Work out the finished part from the listing and answer in its coordinate system (mm). A direction names the side the tool comes from. Coordinates: 2 decimals unless noted, no trailing zeros. Order: outer loops, then holes, each group sorted by start corner. A loop starts at its lowest first (then second) coordinate and runs counter-clockwise, first axis right, second up. Notation, with made-up numbers: (64, -17.5) -> (123, -17.5) arc R12 ccw to (123, 2.5) -> close; hole circle Ø4 at (-27.75, 16). An arc over 180 degrees is marked (long way). Use one line per item in the form item = value.
Autodesk Inventor part; units mm, degrees
ref_plane "YZ Plane" through (0, 0, 0) normal (1, 0, 0) x (0, 1, 0)
ref_plane "XZ Plane" through (0, 0, 0) normal (0, 1, 0) x (-1, 0, 0)
ref_plane "XY Plane" through (0, 0, 0) normal (0, 0, 1) x (1, 0, 0)
sketch "Sketch1: base" plane through (0, 0, 0) normal (0, 0, 1) x (1, 0, 0)
  circle A0 centre (0, 0) radius 18
  line L0 (4.45, -17.4413) -> (4.45, -27.4413)
  line L1 (4.45, -27.4413) -> (-4.45, -27.4413)
  line L2 (-4.45, -27.4413) -> (-4.45, -17.4413)
  line L3 (-2.45, -22.3413) -> (2.45, -22.3413)
  line L4 (2.45, -22.3413) -> (2.45, -25.4413)
  line L5 (2.45, -25.4413) -> (-2.45, -25.4413)
  line L6 (-2.45, -25.4413) -> (-2.45, -22.3413)
  line L7 (-2, -22.2913) -> (2, -22.2913) construction
  line L8 (2, -25.4913) -> (-2, -25.4913) construction
  arc A1 (-2, -22.2913) -> (-2, -25.4913) centre (-0.0791, -23.8913) ccw construction
  arc A2 (2, -25.4913) -> (2, -22.2913) centre (0.0791, -23.8913) ccw construction
  point P0 (0, -22.3413)
  point P1 (0, -27.4413)
  point P2 (0, -22.2913)
  point P3 (-2.45, -23.8913)
  dimension "door_diameter" = 36
  dimension "axle_width" = 4.9
  dimension "axle_height" = 3.1
  dimension "handle_height" = 10
  dimension "spacing_height" = 2
  dimension "spacing_width" = 2
  dimension "d14" = 4
  dimension "d16" = 3.2
  dimension "d17" = 2.5
sketch "Sketch2: text" plane through (0, 0, 0) normal (0, 0, 1) x (1, 0, 0)
  line L0 (-1.5, -16.3413) -> (1.5, -16.3413) construction
  line L1 (1.5, -16.3413) -> (1.5, -19.3413) construction
  line L2 (1.5, -19.3413) -> (-1.5, -19.3413) construction
  line L3 (-1.5, -19.3413) -> (-1.5, -16.3413) construction
  line L4 (4.45, -27.4413) -> (-4.45, -27.4413) construction
  line L5 (-4.45, -27.4413) -> (-4.45, -17.4413) construction
  line L6 (4.45, -17.4413) -> (4.45, -27.4413) construction
  line L7 (-2.45, -22.3413) -> (2.45, -22.3413) construction
  line L8 (2.45, -22.3413) -> (2.45, -25.4413) construction
  line L9 (-2.45, -25.4413) -> (-2.45, -22.3413) construction
  line L10 (2.45, -25.4413) -> (-2.45, -25.4413) construction
  circle A0 centre (0, 0) radius 18 construction
  line L11 (-2.7183, -17.1558) -> (-1.8376, -17.1558)
  line L12 (-1.8376, -17.1558) -> (-1.4061, -18.5561)
  line L13 (-1.4061, -18.5561) -> (-0.9628, -17.1558)
  line L14 (-0.9628, -17.1558) -> (-0.1086, -17.1558)
  line L15 (-0.1086, -17.1558) -> (-1.048, -19.3663)
  line L16 (-1.048, -19.3663) -> (-1.7995, -19.3663)
  line L17 (-1.7995, -19.3663) -> (-2.7183, -17.1558)
  line L18 (0.8777, -17.1969) -> (0.0763, -17.0531)
  spline S0 degree 2 poles (0.0763, -17.0531) (0.1761, -16.6715) (0.7427, -16.2634) (1.2623, -16.2634) knots 0 0 0 1 2 2 2
  spline S1 degree 2 poles (1.2623, -16.2634) (1.8611, -16.2634) (2.3924, -16.7096) (2.3924, -17.0443) knots 0 0 0 1 2 2 2
  spline S2 degree 2 poles (2.3924, -17.0443) (2.3924, -17.2439) (2.1752, -17.5639) (1.9551, -17.6842) knots 0 0 0 1 2 2 2
  spline S3 degree 2 poles (1.9551, -17.6842) (2.1341, -17.7282) (2.2281, -17.787) knots 0 0 0 1 1 1
  spline S4 degree 2 poles (2.2281, -17.787) (2.3807, -17.8809) (2.548, -18.1862) (2.548, -18.3975) knots 0 0 0 1 2 2 2
  spline S5 degree 2 poles (2.548, -18.3975) (2.548, -18.6647) (2.2692, -19.1549) (1.7466, -19.4191) (1.318, -19.4191) knots 0 0 0 1 2 3 3 3
  spline S6 degree 2 poles (1.318, -19.4191) (0.9041, -19.4191) (0.4227, -19.2224) (0.1115, -18.8467) (0.0294, -18.5619) knots 0 0 0 1 2 3 3 3
  line L19 (0.0294, -18.5619) -> (0.8777, -18.4504)
  spline S7 degree 2 poles (0.8777, -18.4504) (0.9276, -18.7058) (1.136, -18.9024) (1.2975, -18.9024) knots 0 0 0 1 2 2 2
  spline S8 degree 2 poles (1.2975, -18.9024) (1.4678, -18.9024) (1.6938, -18.6529) (1.6938, -18.4445) knots 0 0 0 1 2 2 2
  spline S9 degree 2 poles (1.6938, -18.4445) (1.6938, -18.2302) (1.4766, -17.9983) (1.2887, -17.9983) knots 0 0 0 1 2 2 2
  spline S10 degree 2 poles (1.2887, -17.9983) (1.1889, -17.9983) (1.0157, -18.0482) knots 0 0 0 1 1 1
  line L20 (1.0157, -18.0482) -> (1.0597, -17.4406)
  spline S11 degree 2 poles (1.0597, -17.4406) (1.1302, -17.4523) (1.1683, -17.4523) knots 0 0 0 1 1 1
  spline S12 degree 2 poles (1.1683, -17.4523) (1.3357, -17.4523) (1.5588, -17.2409) (1.5588, -17.0942) knots 0 0 0 1 2 2 2
  spline S13 degree 2 poles (1.5588, -17.0942) (1.5588, -16.9562) (1.3914, -16.7889) (1.2476, -16.7889) knots 0 0 0 1 2 2 2
  spline S14 degree 2 poles (1.2476, -16.7889) (1.0979, -16.7889) (0.91, -16.9709) (0.8777, -17.1969) knots 0 0 0 1 2 2 2
  point P0 (0, -19.3413)
  point P1 (0, -22.3413)
  dimension "x_t2" = 3
  dimension "x_t3" = 3
extrude "Ex1: base" add sketch "Sketch1: base" against normal blind 2
extrude "Ex2: text" cut sketch "Sketch2: text" against normal blind 0.5
fillet "Fillet1" radius 2 4 edges at (4.45, -17.4413, -1) (-4.45, -17.4413, -1) (4.45, -27.4413, -1) (-4.45, -27.4413, -1)
fillet "Fillet2" [suppressed]
properties part number "door_03"
(1) This flat-tipped pin is pushed along its axis until it touches: P1, Ø0.6, axis at x = -1.5, z = 0, coming from the +Y side. Where does it stop, or does it pass through?
Data:
P1 = 17.96
(2) Section C-C on y = 5 is taken. Write down the section's boundary in (x, z), plus the area to 3 significant figures.
Data:
outline = (-17.29, -2) -> (17.29, -2) -> (17.29, 0) -> (-17.29, 0) -> close
area = 69.2 mm²
(3) Section B-B on x = -10 is taken. Write down the section's boundary in (y, z), plus the area to 3 significant figures.
Data:
outline = (-14.97, -2) -> (14.97, -2) -> (14.97, 0) -> (-14.97, 0) -> close
area = 59.9 mm²
(4) Section A-A on z = -0.95 is taken. Write down the section's boundary in (x, y) (3 decimals), plus the area to 3 significant figures.
Data:
outline = (-5.805, -17.038) arc R2 cw to (-4.45, -18.931) -> (-4.45, -25.441) arc R2 ccw to (-2.45, -27.441) -> (2.45, -27.441) arc R2 ccw to (4.45, -25.441) -> (4.45, -18.931) arc R2 cw to (5.805, -17.038) arc R18 ccw (long way) to start; hole (-2.45, -25.441) -> (2.45, -25.441) -> (2.45, -22.341) -> (-2.45, -22.341) -> close
area = 1,090 mm²
(5) The mould has two halves that part along X. Classify faces 1 (the cylindrical face through (4.8, -17.8, -1)), 2 (the flat face through (2.45, -24, -1)), 3 (the flat face through (0, 1, 0)), 4 (the cylindrical face through (-3.85, -26.87, -1.01)): released by +X, released by -X, zero draft, split by the parting line, or undercut.
Data:
face_1 = released by +X
face_2 = undercut
face_3 = zero draft
face_4 = released by -X
(6) Which of the six approach directions +Z, -Z, +X, -X, +Y, -Y give full straight-line access (tool end or side, diameter ignored) to faces 5 (the flat face through (-1, -18, -0.5)), 6 (the flat face through (-4.45, -22, -1)), 7 (the flat face through (0, -22.341, -1)), 8 (the flat face through (0, -27.441, -1)), 9 (the flat face through (4.45, -22, -1))?
Data:
face_5 = +Z
face_6 = +Z, -Z, -X, -Y
face_7 = +Z, -Z
face_8 = +Z, -Z, +X, -X, -Y
face_9 = +Z, -Z, +X, -Y
(7) Straight lines are drawn through the part: line 1 along Y through (x, z) = (0, -1.45); line 2 along X through (y, z) = (-19, -1.3); line 3 along X through (y, z) = (-0.5, -1.4). For each, find the intervals that lie inside material, in ascending order.
Data:
line_1 = -27.44 to -25.44, -22.34 to 18
line_2 = -4.45 to 4.45
line_3 = -17.99 to 17.99
